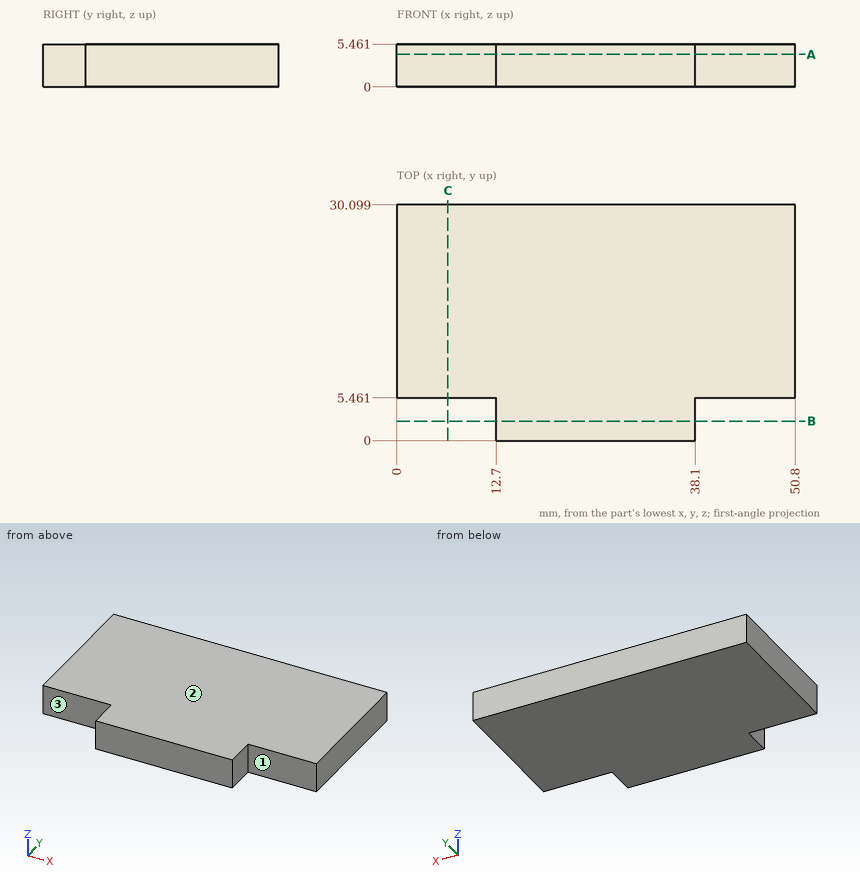
Print and shaded views of the part. All mm, measured from the part's lowest x, y and z. A direction names the side the tool comes from. Give positions to 0.01 mm unless a question says otherwise; leave off trailing zeros. Loops run counter-clockwise (first coordinate to the right, second up) from the corner with the lowest first, then second, coordinate; pieces in that order, holes last.
1) Saw through at A-A (z = 4.15). Write the cut outline in (x, y), plus the area to 3 significant figures.
2) Wall check: line 1 (Y direction, x = 44, z = 3.05); line 2 (X direction, y = 3, z = 4). Give the ranges that are in metal, low to high.
3) Saw through at C-C (x = 6.5). Write the cut outline in (y, z).
4) Tool access for the marked faces 1, 2 and 3: list every direction of +Z, -Z, +X, -X, +Y, -Y with a clear straight run to the whole face (end or side of a thin tool).
5) Saw through at B-B (y = 2.5). Write the cut outline in (x, z), plus the area to 3 significant figures.
6) Flat gauge pin, fed straight in: pin 1 Ø1.6 at (y, z) = (2.5, 3) entering from -X. Where does the tip first touch, or does it go through?
Answer block:
1. outline: (0, 5.46) - (12.7, 5.46) - (12.7, 0) - (38.1, 0) - (38.1, 5.46) - (50.8, 5.46) - (50.8, 30.1) - (0, 30.1) - close
1. area: 1,390 mm2
2. line 1: y = 5.46 to 30.1
2. line 2: x = 12.7 to 38.1
3. outline: (5.46, 0) - (30.1, 0) - (30.1, 5.46) - (5.46, 5.46) - close
4. face 1: +Z, -Z, +X, -Y
4. face 2: +Z, +X, -X, +Y, -Y
4. face 3: +Z, -Z, -X, -Y
5. outline: (12.7, 0) - (38.1, 0) - (38.1, 5.46) - (12.7, 5.46) - close
5. area: 139 mm2
6. pin 1: stops at x = 12.7
